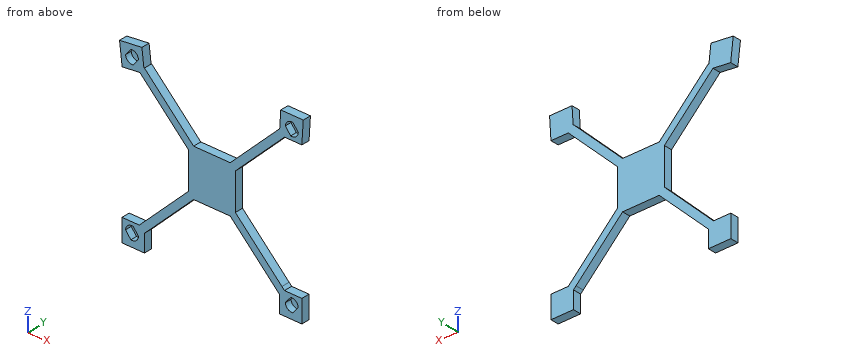
from build123d import *

# Parameters (mm, degrees)
BOSS_EXTRUDE1_DEPTH = 12.7
BOSS_EXTRUDE6_DEPTH = 12.7
CUT_EXTRUDE1_DEPTH  = 10


with BuildPart() as part:
    # Sketch1 → Boss-Extrude1 (new body)
    with BuildSketch(Plane(origin=(0, 0, 0), x_dir=(1, 0, 0), z_dir=(0, 1, 0))):
        Polygon((0, 0), (-71.842048969, 71.842048969), (-63.880459669, 79.803638268), (7.961589299, 7.961589299), (64.406033744, 7.961589299), (136.248082712, 79.803638268), (144.209672011, 71.842048969), (72.367623043, 0), (72.367623043, -56.444444444), (144.209672011, -128.286493413), (136.248082712, -136.248082712), (64.406033744, -64.406033744), (7.961589299, -64.406033744), (-63.880459669, -136.248082712), (-71.842048969, -128.286493413), (0, -56.444444444), align=None)
    extrude(amount=BOSS_EXTRUDE1_DEPTH)

    # Sketch4 → Boss-Extrude6 (add)
    with BuildSketch(Plane(origin=(0, 12.7, 0), x_dir=(1, 0, 0), z_dir=(0, 1, 0))):
        Polygon((-67.861254319, 110.511019008), (-102.549429709, 110.511019008), (-102.549429709, 75.822843618), (-75.822843618, 75.822843618), (-67.904353545, 83.741333692), (-67.861254319, 83.698234466), align=None)
        Polygon((-63.923558895, 79.760539042), (-67.861254319, 83.698234466), (-67.861254319, 75.822843618), align=None)
        Polygon((-67.861254319, 75.822843618), (-67.861254319, 83.698234466), (-67.904353545, 83.741333692), (-75.822843618, 75.822843618), align=None)
        Polygon((-67.861254319, 75.822843618), (-75.822843618, 75.822843618), (-71.842048969, 71.842048969), align=None)
        Polygon((148.06163561, 75.822843618), (140.228877362, 75.822843618), (140.228877362, 83.741333692), (136.248082712, 79.803638268), (144.168507311, 71.79652231), (148.14930196, 75.734217734), align=None)
        Polygon((140.228877362, 83.741333692), (140.228877362, 75.822843618), (148.06163561, 75.822843618), align=None)
        Polygon((140.228877362, 110.511019008), (140.228877362, 83.741333692), (148.06163561, 75.822843618), (174.917052842, 75.822843618), (174.917052842, 110.511019008), align=None)
        Polygon((144.209672011, -128.286493413), (140.228877362, -132.267288063), (147.887031193, -132.267288063), (148.038748927, -132.115570329), align=None)
        Polygon((147.887031193, -132.267288063), (140.228877362, -132.267288063), (140.680194952, -139.474124303), align=None)
        Polygon((140.680194952, -139.474124303), (140.228877362, -132.267288063), (136.248082712, -136.248082712), (140.077159628, -140.077159628), align=None)
        Polygon((174.917052842, -132.267288063), (147.887031193, -132.267288063), (140.680194952, -139.474124303), (142.396926606, -166.887644511), (177.085102086, -166.887644511), align=None)
        Polygon((-63.880459669, -136.248082712), (-67.861254319, -132.267288063), (-68.687385193, -139.452020723), (-67.885891437, -140.25351448), align=None)
        Polygon((-68.687385193, -139.452020723), (-67.861254319, -132.267288063), (-75.001794215, -131.446238659), (-75.847480736, -132.29192518), align=None)
        Polygon((-75.001794215, -131.446238659), (-67.861254319, -132.267288063), (-71.842048969, -128.286493413), align=None)
        Polygon((-71.823738367, -166.728400034), (-68.687385193, -139.452020723), (-75.847480736, -132.29192518), (-75.001794215, -131.446238659), (-102.32236629, -128.304804015), (-106.284850338, -162.765915986), align=None)
    extrude(amount=-BOSS_EXTRUDE6_DEPTH)

    # Sketch10 → Cut-Extrude1 (cut)
    with BuildSketch(Plane(origin=(0, 0, 0), x_dir=(-1, 0, 0), z_dir=(0, -1, 0))):
        with BuildLine():
            ThreePointArc((77.08647461, 91.590101085), (80.856009684, 98.904678295), (88.835255683, 100.915665051))
            Line((88.835255683, 100.915665051), (97.059630047, 90.554214075))
            ThreePointArc((97.059630047, 90.554214075), (93.290094973, 83.239636865), (85.310848974, 81.228650109))
            Line((85.310848974, 81.228650109), (77.08647461, 91.590101085))
        make_face()
        with BuildLine():
            Line((-169.42725309, 90.554214075), (-161.202878726, 100.915665051))
            ThreePointArc((-161.202878726, 100.915665051), (-153.223632727, 98.904678295), (-149.454097653, 91.590101085))
            Line((-149.454097653, 91.590101085), (-157.678472017, 81.228650109))
            ThreePointArc((-157.678472017, 81.228650109), (-165.657718016, 83.239636865), (-169.42725309, 90.554214075))
        make_face()
        with BuildLine():
            ThreePointArc((-149.454097653, -148.034545529), (-153.223632727, -155.34912274), (-161.202878726, -157.360109496))
            Line((-161.202878726, -157.360109496), (-169.42725309, -146.99865852))
            ThreePointArc((-169.42725309, -146.99865852), (-165.657718016, -139.684081309), (-157.678472017, -137.673094553))
            Line((-157.678472017, -137.673094553), (-149.454097653, -148.034545529))
        make_face()
        with BuildLine():
            ThreePointArc((77.08647461, -148.034545529), (80.856009684, -155.34912274), (88.835255683, -157.360109496))
            Line((88.835255683, -157.360109496), (97.059630047, -146.99865852))
            ThreePointArc((97.059630047, -146.99865852), (93.290094973, -139.684081309), (85.310848974, -137.673094553))
            Line((85.310848974, -137.673094553), (77.08647461, -148.034545529))
        make_face()
    extrude(amount=-CUT_EXTRUDE1_DEPTH, mode=Mode.SUBTRACT)


solid = part.part
Geometry: final body of the model. Coordinates: model frame, mm. Give positions to 0.01 mm unless a question says otherwise; leave off trailing zeros. Loops run counter-clockwise (first coordinate to the right, second up) from the corner with the lowest first, then second, coordinate; pieces in that order, holes last. Notation, with made-up numbers: M 76.25,84 L 84.25,84 A16 cw 84.25,88 Z; hole C 29.5,33 d3. An arc over 180 degrees is marked long. Put each result on its own line as item: value.
1) Cut plane D-D, the plane x = 40.5. Return the cut outline in (y, z).
Computed values:
outline: M 0,-7.96 L 12.7,-7.96 L 12.7,64.41 L 0,64.41 Z
2) Cut plane C-C, the plane y = 7.5. Give the number of separate pieces and of enclosed holes in the cut face, plus the area to 3 significant figures.
Computed values:
separate pieces: 1
enclosed holes: 4
area: 13,500 mm^2
3) Cut plane B-B, the plane x = 99.5. Return the cut outline in (y, z), plus the area to 3 significant figures.
Computed values:
outline: M 0,-43.06 L 12.7,-43.06 L 12.7,-27.13 L 0,-27.13 Z; M 0,83.58 L 12.7,83.58 L 12.7,99.5 L 0,99.5 Z
area: 404 mm^2
4) Material intervals for L1, parallel to Z at x = -88.5, y = 7; L2, parallel to Z at x = 10, y = 1.5; L3, parallel to Z at x = 86.5, y = 7.25, sorted ascending. Write a range as from..to.
Computed values:
L1: z = -110.51..-100.97, -81.17..-75.82, 129.89..137.62, 157.41..164.81
L2: z = -7.96..64.41
L3: z = -30.06..-14.13, 70.58..86.5
5) Cut plane A-A, the plane z = 91.5. Return the cut outline in (x, y).
Computed values:
outline: M -35.06,0 L -19.13,0 L -19.13,12.7 L -35.06,12.7 Z; M 91.5,0 L 107.42,0 L 107.42,12.7 L 91.5,12.7 Z
6) First-contact query: P1, Ø4, axis at y = 8, z = -90.5, coming from the -X side; P2, Ø1.5, axis at x = -31, y = 8.5, coming from the +Z side; P3, Ø6, axis at x = 158.5, z = -87, coming from the -Y side. Flat tips, straight axial feed; report the tip coordinate or a pass-through.
Computed values:
P1: stops at x = -102.55
P2: stops at z = 104.12
P3: stops at y = 10
